Read the model definition and answer for the solid it produces. Units are mm, in the model's axes. A direction names the side the tool comes from. Coordinates: 2 decimals unless noted, no trailing zeros. Write each loop counter-clockwise with the first axis right and the second up, starting at its lowest first coordinate (ties: lowest second). Pieces come first, ordered by that corner, then holes. Notation, with made-up numbers: M 40,43 L 89,43 A21 ccw 89,77 Z; hole C -14.5,-28.75 d9. An arc over 180 degrees is marked long. Use a Markdown table: item, result. Add a question column.
from build123d import *

# Parameters (mm, degrees)
CUT_EXTRUDE2_DEPTH      = 22
CUT_EXTRUDE2_DEPTH_BACK = 21
SKETCH2_R               = 3
SKETCH3_R               = 3
CUT_EXTRUDE3_DEPTH      = 45


with BuildPart() as part:
    # Sketch1 → Revolve1 (revolve)
    with BuildSketch(Plane.XY, mode=Mode.PRIVATE) as revolve1_sk:
        Polygon((-40, 0), (40, 0), (40, 5), (39, 6), (25, 6), (25, 9), (-25, 9), (-25, 6), (-39, 6), (-40, 5), align=None)
    revolve(revolve1_sk.sketch.rotate(Axis((-40, 0, 0), (1, 0, 0)), 90), axis=Axis((-40, 0, 0), (1, 0, 0)))

    # Sketch2 → Cut-Extrude2 (cut, two sides: drawn at the far end of the back side and taken through both)
    with BuildSketch(Plane.XY.offset(-CUT_EXTRUDE2_DEPTH_BACK)):
        with Locations(Location((0, 0, 0), (0, 0, 180))):
            Circle(SKETCH2_R)
    extrude(amount=CUT_EXTRUDE2_DEPTH + CUT_EXTRUDE2_DEPTH_BACK, mode=Mode.SUBTRACT)

    # Sketch3 → Cut-Extrude3 (cut)
    with BuildSketch(Plane(origin=(40, 0, 0), x_dir=(0, 0, -1), z_dir=(1, 0, 0))):
        Circle(SKETCH3_R)
    extrude(amount=-CUT_EXTRUDE3_DEPTH, mode=Mode.SUBTRACT)


solid = part.part
Item 1: Find section A-A on y = 0. Give the vertices of the cut face in (x, z).
Item 2: For faces 4 (the flat face through (-40, 0, 0)), 5 (the cylindrical face through (20, 0, 3)), determine the directions among +Z, -Z, +X, -X, +Y, -Y from which every point of the face is accessible in a straight line to the end or side of a thin tool.
Item 3: Find section D-D on x = -29. Give the vertices of the cut face in (y, z), then the cut area to 3 significant figures.
Item 4: Consider probe 1 along Y at (x, z) = (-2.4, 0); probe 2 along X at (y, z) = (-1.75, 2); probe 3 along X at (y, z) = (-5.5, -5.25). Determine where each line is inside the solid, lowest interval first.
Item 5: Find section B-B on x = 7.5. Give the vertices of the cut face in (y, z).
Item 6: Each of these flat-tipped pins is pushed along its axis until it touches: pin 1 (2 mm diameter, centred on y = 1.5, z = 0.5, fed in from +X); pin 2 (5.5 mm diameter, centred on x = 0, y = 0, fed in from +Z); pin 3 (1.5 mm diameter, centred on x = 12.5, z = -5, fed in from +Y). Where does it stop, or does it pass through?
Item 7: Determine the mould class of faces 1 (the cylindrical face through (-32.098, -1.802, 5.723)), 2 (the flat face through (-25, 6, 2)), 3 (the cylindrical face through (3, 0, -6)) for opening direction Y: pulls with the +Y half, pulls with the -Y half, needs draft (parallel to the pull), parting line crosses it, or undercut.
Item 8: Find section C-C on x = -8. Give the vertices of the cut face in (y, z), then the cut area to 3 significant figures.
Geometry says:
| question | item | result |
|---|---|---|
| 1 | outline | M -40,-5 L -39,-6 L -25,-6 L -25,-9 L -3,-9 L -3,-3 L -5,-3 L -5,3 L -3,3 L -3,9 L -25,9 L -25,6 L -39,6 L -40,5 Z; M 3,-9 L 25,-9 L 25,-6 L 39,-6 L 40,-5 L 40,-3 L 3,-3 Z; M 3,3 L 40,3 L 40,5 L 39,6 L 25,6 L 25,9 L 3,9 Z |
| 2 | face 4 | +Z, -Z, -X, +Y, -Y |
| 2 | face 5 | +X |
| 3 | outline | C 0,0 d12 |
| 3 | area | 113 mm2 |
| 4 | probe 1 | y = -9 to -3, 3 to 9 |
| 4 | probe 2 | x = -40 to -5 |
| 4 | probe 3 | x = -25 to 25 |
| 5 | outline | C 0,0 d18; hole C 0,0 d6 |
| 6 | pin 1 | stops at x = -5 |
| 6 | pin 2 | passes through |
| 6 | pin 3 | stops at y = 7.93 |
| 7 | face 1 | parting line crosses it |
| 7 | face 2 | needs draft |
| 7 | face 3 | undercut |
| 8 | outline | C 0,0 d18 |
| 8 | area | 254 mm2 |
